Check sheet for the modelled part. Datum: model origin and axes. Units: mm. Face numbers are marked on the shaded views. Round coordinates to 2 decimals unless told otherwise and drop trailing zeros. Write each loop counter-clockwise with the first axis right and the second up, starting at its lowest first coordinate (ties: lowest second). Pieces come first, ordered by that corner, then holes. Notation, with made-up numbers: M -3,4 L 18,4 A18 ccw 18,15 Z; hole C 60.5,14 d8. An arc over 180 degrees is marked long. Put each result on its own line as item: value.
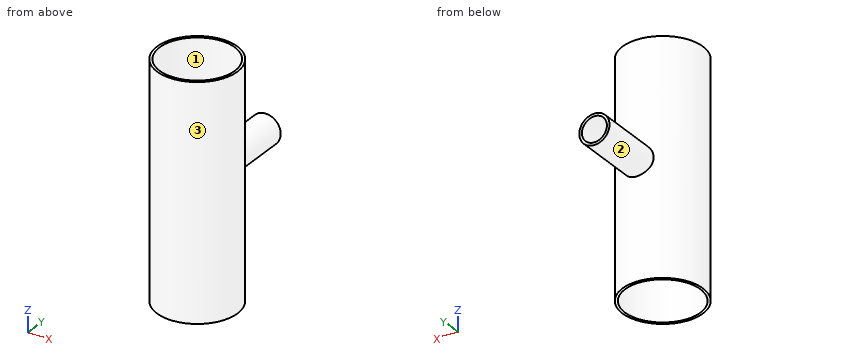
Autodesk Inventor part; units mm, degrees
ref_plane "YZ Plane" through (0, 0, 0) normal (1, 0, 0) x (0, 1, 0)
ref_plane "XZ Plane" through (0, 0, 0) normal (0, 1, 0) x (-1, 0, 0)
ref_plane "XY Plane" through (0, 0, 0) normal (0, 0, 1) x (1, 0, 0)
sketch "Sketch1" plane through (0, 0, 0) normal (0, 0, 1) x (1, 0, 0)
  circle A0 centre (0, 0) radius 25.4
  dimension "d0" = 50.8
extrude "Extrusion1" add sketch "Sketch1" along normal mid plane 146
sketch "Sketch2" plane through (0, 0, 0) normal (0, 1, 0) x (-1, 0, 0)
  circle A0 centre (0, 0) radius 9.525
  dimension "d3" = 19.05
extrude "Extrusion2" add sketch "Sketch2" along normal blind 66.5
shell "Shell1" thickness 1.65 removed faces 3 at (2.8113, 66.5, 0.0442) at (-7.2508, -1.9085, 73) at (-7.2508, -1.9085, -73)
properties part number "ASME BPE - RED TEE-50.8-19.05" material "Stainless Steel, 316L"
1. Cross-section at A-A (y = 0). Enter the section's corners in (x, z).
Computed values:
outline: M -25.4,-73 L -23.75,-73 L -23.75,73 L -25.4,73 Z; M 23.75,-73 L 25.4,-73 L 25.4,73 L 23.75,73 Z
2. Cross-section at B-B (x = 0). Enter the section's corners in (y, z) (3 decimals), then the cut area to 3 significant figures.
Computed values:
outline: M -25.4,-73 L -23.75,-73 L -23.75,73 L -25.4,73 Z; M 23.75,-73 L 25.4,-73 L 25.4,-9.525 L 66.5,-9.525 L 66.5,-7.875 L 23.75,-7.875 Z; M 23.75,7.875 L 66.5,7.875 L 66.5,9.525 L 25.4,9.525 L 25.4,73 L 23.75,73 Z
area: 591 mm2
3. Depth check by flat-ended pin: pin 1 Ø8 at (x, y) = (5, 44.5) entering from -Z; pin 2 Ø6 at (y, z) = (14, 16.5) entering from -X; pin 3 Ø10 at (y, z) = (-12, 14) entering from -X. Enter the tip coordinate at first touch or a pass-through.
Computed values:
pin 1: stops at z = -9.47
pin 2: stops at x = -22.89
pin 3: stops at x = -24.42
4. Cross-section at D-D (x = 19). Enter the section's corners in (y, z).
Computed values:
outline: M -16.86,-73 L -14.25,-73 L -14.25,73 L -16.86,73 Z; M 14.25,-73 L 16.86,-73 L 16.86,73 L 14.25,73 Z
5. Scan lines: probe 1 along Z at (x, y) = (0, 33) (3 decimals); probe 2 along Y at (x, z) = (0, -23). Record each from-to range of solid material in increasing order.
Computed values:
probe 1: z = -9.525 to -7.875, 7.875 to 9.525
probe 2: y = -25.4 to -23.75, 23.75 to 25.4
6. Release check for a two-part mould opening along Y. For the marked faces 1, 2 and 3 record: +Y half, -Y half, draft (parallel to the pull), parting line (faces both ways), or undercut.
Computed values:
face 1: undercut
face 2: draft
face 3: parting line
7. Cross-section at C-C (z = 0). Enter the section's corners in (x, y) (3 decimals), then the cut area to 3 significant figures.
Computed values:
outline: M -9.525,23.546 A25.4 ccw long 9.525,23.546 L 9.525,66.5 L 7.875,66.5 L 7.875,22.406 A23.75 cw long -7.875,22.406 L -7.875,66.5 L -9.525,66.5 Z
area: 369 mm2
